Geometry: final body of the model. Coordinates: model frame, mm. Round coordinates to 2 decimals unless told otherwise and drop trailing zeros. One line per item, written item: value. Start each with the question number.
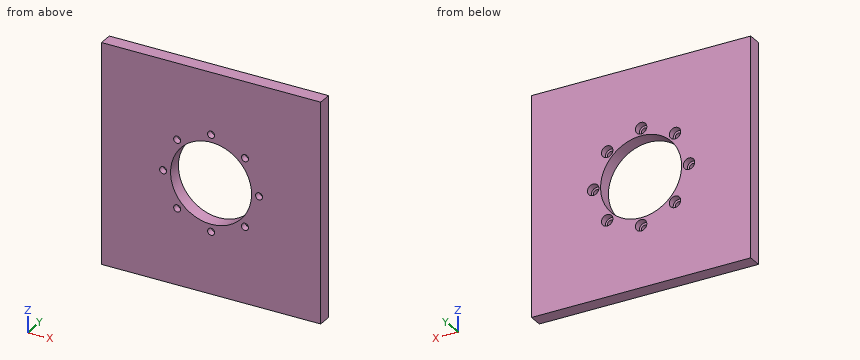
from build123d import *

# Parameters (mm, degrees)
SKETCH1_W                                        = 304.8
SKETCH1_H                                        = 304.8
SKETCH1_R                                        = 56.35625
BOSS_EXTRUDE1_DEPTH                              = 19.05
CBORE_FOR_3_8_SOCKET_HEAD_CAP_SCREW1_D           = 9.8044
CBORE_FOR_3_8_SOCKET_HEAD_CAP_SCREW1_CBORE_D     = 15.875
CBORE_FOR_3_8_SOCKET_HEAD_CAP_SCREW1_CBORE_DEPTH = 9.525


with BuildPart() as part:
    # Sketch1 → Boss-Extrude1 (new body)
    with BuildSketch(Plane(origin=(0, 0, 0), x_dir=(1, 0, 0), z_dir=(0, 1, 0))):
        Rectangle(SKETCH1_W, SKETCH1_H)
        with Locations(Location((0, 0, 0), (0, 0, 90))):
            Circle(SKETCH1_R, mode=Mode.SUBTRACT)
    extrude(amount=BOSS_EXTRUDE1_DEPTH)

    # CBORE for 3/8 Socket Head Cap Screw1 (through all)
    with Locations(Plane(origin=(0, 19.05, 0), x_dir=(1, 0, 0), z_dir=(0, 1, 0))):
        with Locations((47.146344636, -47.146344636), (66.675, 0), (47.146344636, 47.146344636), (0, 66.675), (-47.146344636, 47.146344636), (-66.675, 0), (-47.146344636, -47.146344636), (0, -66.675)):
            CounterBoreHole(CBORE_FOR_3_8_SOCKET_HEAD_CAP_SCREW1_D / 2, CBORE_FOR_3_8_SOCKET_HEAD_CAP_SCREW1_CBORE_D / 2, CBORE_FOR_3_8_SOCKET_HEAD_CAP_SCREW1_CBORE_DEPTH)


solid = part.part
(1) Section query A-A (z = 0). Count the separate pieces of the cut face and the enclosed holes in it, and give its area (3 significant figures).
(2) Pin query (flat end, axial travel): pin 1 (12.5 mm diameter, centred on x = 47.15, z = -47.15, fed in from +Y) (3 decimals). Return the tip coordinate at first contact, or that it passes through.
(3) Line query: probe 1 along X at (y, z) = (4.5, -48.5); probe 2 along X at (y, z) = (14.5, 6); probe 3 along Z at (x, y) = (41, 15.5). Output: solid intervals per line, ascending.
Results list:
1. separate pieces: 4
1. enclosed holes: 0
1. area: 3,170 mm^2
2. pin 1: stops at y = 9.525
3. probe 1: x = -152.4 to -51.86, -42.43 to -28.7, 28.7 to 42.43, 51.86 to 152.4
3. probe 2: x = -152.4 to -71.87, -61.48 to -56.04, 56.04 to 61.48, 71.87 to 152.4
3. probe 3: z = -152.4 to -52.17, -42.12 to -38.67, 38.67 to 42.12, 52.17 to 152.4
